Geometry check sheet. Reference: the model listing, model coordinates, mm. Face numbers are marked on the shaded views. A direction names the side the tool comes from. Round coordinates to 2 decimals unless told otherwise and drop trailing zeros. Order: outer loops, then holes, each group sorted by start corner. A loop starts at its lowest first (then second) coordinate and runs counter-clockwise, first axis right, second up.
Autodesk Inventor part; units mm, degrees
ref_plane "YZ Plane" through (0, 0, 0) normal (1, 0, 0) x (0, 1, 0)
ref_plane "XZ Plane" through (0, 0, 0) normal (0, 1, 0) x (-1, 0, 0)
ref_plane "XY Plane" through (0, 0, 0) normal (0, 0, 1) x (1, 0, 0)
sketch "Sketch1" plane through (0, 0, 0) normal (0, 1, 0) x (-1, 0, 0)
  line L0 (0, 0) -> (57.023, 0)
  line L1 (57.023, 0) -> (57.023, -24.765)
  line L2 (57.023, -24.765) -> (0, -24.765)
  line L3 (0, -24.765) -> (0, 0)
  dimension "d0" = 57.023
  dimension "d1" = 24.765
extrude "Extrusion1" add sketch "Sketch1" along normal blind 3.175
sketch "Sketch3" plane through (0, 0, 0) normal (0, -1, 0) x (1, 0, 0)
  line L0 (-3.175, -3.175) -> (-15.113, -3.175)
  line L1 (-15.113, -3.175) -> (-15.113, -21.59)
  line L2 (-15.113, -21.59) -> (-3.175, -21.59)
  line L3 (-3.175, -21.59) -> (-3.175, -3.175)
  line L4 (0, -24.765) -> (0, 0)
  line L5 (-57.023, 0) -> (0, 0)
  dimension "d18" = 18.415
  dimension "d19" = 11.938
  dimension "d20" = 3.175
  dimension "d21" = 3.175
extrude "Extrusion3" add sketch "Sketch3" along normal blind 2.921
fillet "Fillet2" radius 1.5875 4 edges at (0, 1.5875, -24.765) (0, 1.5875, 0) (-57.023, 1.5875, 0) (-57.023, 1.5875, -24.765)
hole "Hole2" at (-9.144, -2.921, -12.3825) direction (0, 1, 0) diameter 10.16 depth 25.4
sketch "Sketch4" plane through (0, 3.175, 0) normal (0, 1, 0) x (1, 0, 0)
  line L0 (-3.8735, 17.653) -> (-14.4145, 17.653)
  line L1 (-14.4145, 17.653) -> (-14.4145, 7.112)
  line L2 (-14.4145, 7.112) -> (-3.8735, 7.112)
  line L3 (-3.8735, 7.112) -> (-3.8735, 17.653)
  line L4 (-1.5875, 24.765) -> (-55.4355, 24.765)
  line L5 (0, 1.5875) -> (0, 23.1775)
  point P0 (0, 0)
  dimension "d34" = 10.541
  dimension "d35" = 10.541
  dimension "d36" = 7.112
  dimension "d37" = 3.8735
extrude "Extrusion4" cut sketch "Sketch4" against normal blind 3.175
sketch "Sketch5" plane through (0, 3.175, 0) normal (0, 1, 0) x (1, 0, 0)
  line L0 (0, 1.5875) -> (0, 23.1775)
  line L1 (-1.9431, 1.5875) -> (-1.9431, 23.1775)
  line L2 (-55.4355, 24.765) -> (-1.5875, 24.765)
  line L3 (-1.5875, 0) -> (-1.9431, 0)
  line L4 (-1.9431, 0) -> (-1.9431, 24.765)
  line L5 (-1.9431, 24.765) -> (-1.5875, 24.765)
  line L6 (0, 23.1775) -> (0, 1.5875)
  arc A0 (0, 23.1775) -> (-1.5875, 24.765) centre (-1.5875, 23.1775) ccw
  arc A1 (-1.5875, 0) -> (0, 1.5875) centre (-1.5875, 1.5875) ccw
  line L7 (-57.023, 23.1775) -> (-57.023, 1.5875)
  line L8 (-55.0672, 23.1775) -> (-55.0672, 1.5875)
  line L9 (-1.5875, 0) -> (-55.4355, 0)
  line L10 (-55.0672, 0) -> (-55.4355, 0)
  line L11 (-57.023, 1.5875) -> (-57.023, 23.1775)
  line L12 (-55.4355, 24.765) -> (-55.0672, 24.765)
  line L13 (-55.0672, 24.765) -> (-55.0672, 0)
  arc A2 (-57.023, 1.5875) -> (-55.4355, 0) centre (-55.4355, 1.5875) ccw
  arc A3 (-55.4355, 24.765) -> (-57.023, 23.1775) centre (-55.4355, 23.1775) ccw
  point P0 (0, 0)
  dimension "d40" = 1.9431
  dimension "d41" = 1.5875
  dimension "d42" = 1.9558
  dimension "d43" = 1.5875
extrude "Extrusion5" add sketch "Sketch5" along normal blind 30.5308 contours A1 L3 L4 L1 L2 A0 L0 | L9 A2 L7 A3 L2 L13 L8
fillet "Fillet3" radius 1.5875 2 edges at (-1.9431, 3.175, -12.3825) (-55.0672, 3.175, -12.3825)
fillet "Fillet4" radius 0.7937 4 edges at (-9.144, 3.175, -7.112) (-14.4145, 3.175, -12.3825) (-3.8735, 3.175, -12.3825) (-9.144, 3.175, -17.653)
properties part number "switch mount"
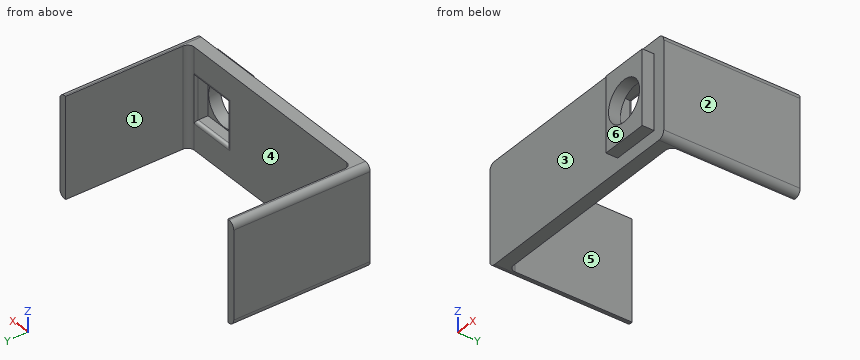
(1) Draft check along X on the marked faces 1, 2, 3 and 4. Enter one of: released by +X, released by -X, zero draft, split by the parting line, or undercut.
Returned:
face 1: undercut
face 2: released by +X
face 3: zero draft
face 4: undercut
(2) Material ranges on line 1 (X direction, y = 31.5, z = -4.75); line 2 (X direction, y = 2.5, z = -8); line 3 (Y direction, x = -1.5, z = -3), recorded low to high.
Returned:
line 1: x = -57.02 to -55.07, -1.94 to 0
line 2: x = -57.02 to -14.42, -3.87 to 0
line 3: y = 0 to 33.71
(3) Sectioned sample at C-C, the plane x = -7. Record the cut outline in (y, z) (3 decimals), and give its area (3 significant figures).
Returned:
outline: (-2.921, -21.59) - (0, -21.59) - (0, -24.765) - (3.175, -24.765) - (3.175, -18.447) arc R0.794 ccw to (2.381, -17.653) - (0, -17.653) - (0, -16.988) - (-2.921, -16.988) - close; (-2.921, -7.777) - (0, -7.777) - (0, -7.112) - (2.381, -7.112) arc R0.794 ccw to (3.175, -6.318) - (3.175, 0) - (0, 0) - (0, -3.175) - (-2.921, -3.175) - close
area: 71.8 mm2
(4) Depth check by flat-ended pin: P1, Ø11.5, axis at x = -11.5, z = -13, coming from the +Y side (3 decimals); P2, Ø7.5, axis at x = -31.5, z = -7.5, coming from the -Y side; P3, Ø0.9, axis at x = -10, y = -2, coming from the +Z side (3 decimals). Enter the tip coordinate at first touch or a pass-through.
Returned:
P1: stops at y = 3.175
P2: stops at y = 0
P3: stops at z = -3.175
(5) Sectioned sample at B-B, the plane z = -9. Record the cut outline in (x, y) (1 decimal).
Returned:
outline: (-57, 0) - (-15.1, 0) - (-15.1, -2.9) - (-12.9, -2.9) - (-12.9, 0) - (-14.4, 0) - (-14.4, 2.4) arc R0.8 ccw to (-15.2, 3.2) - (-53.5, 3.2) arc R1.6 cw to (-55.1, 4.8) - (-55.1, 33.7) - (-57, 33.7) - close; (-5.4, -2.9) - (-3.2, -2.9) - (-3.2, 0) - (0, 0) - (0, 33.7) - (-1.9, 33.7) - (-1.9, 4.8) arc R1.6 cw to (-3.5, 3.2) arc R0.8 ccw to (-3.9, 2.5) - (-3.9, 0) - (-5.4, 0) - close
(6) Set-up check for the marked faces 5 and 6: record each of +Z, -Z, +X, -X, +Y, -Y from which the full face is reachable in a straight line by a thin tool's end or side.
Returned:
face 5: +Z, -Z, +Y
face 6: +Z, -Z, +X, -X, -Y
(7) Sectioned sample at D-D, the plane z = -4.5. Record the cut outline in (x, y) (1 decimal).
Returned:
outline: (-57, 0) - (-15.1, 0) - (-15.1, -2.9) - (-3.2, -2.9) - (-3.2, 0) - (0, 0) - (0, 33.7) - (-1.9, 33.7) - (-1.9, 4.8) arc R1.6 cw to (-3.5, 3.2) - (-53.5, 3.2) arc R1.6 cw to (-55.1, 4.8) - (-55.1, 33.7) - (-57, 33.7) - close
